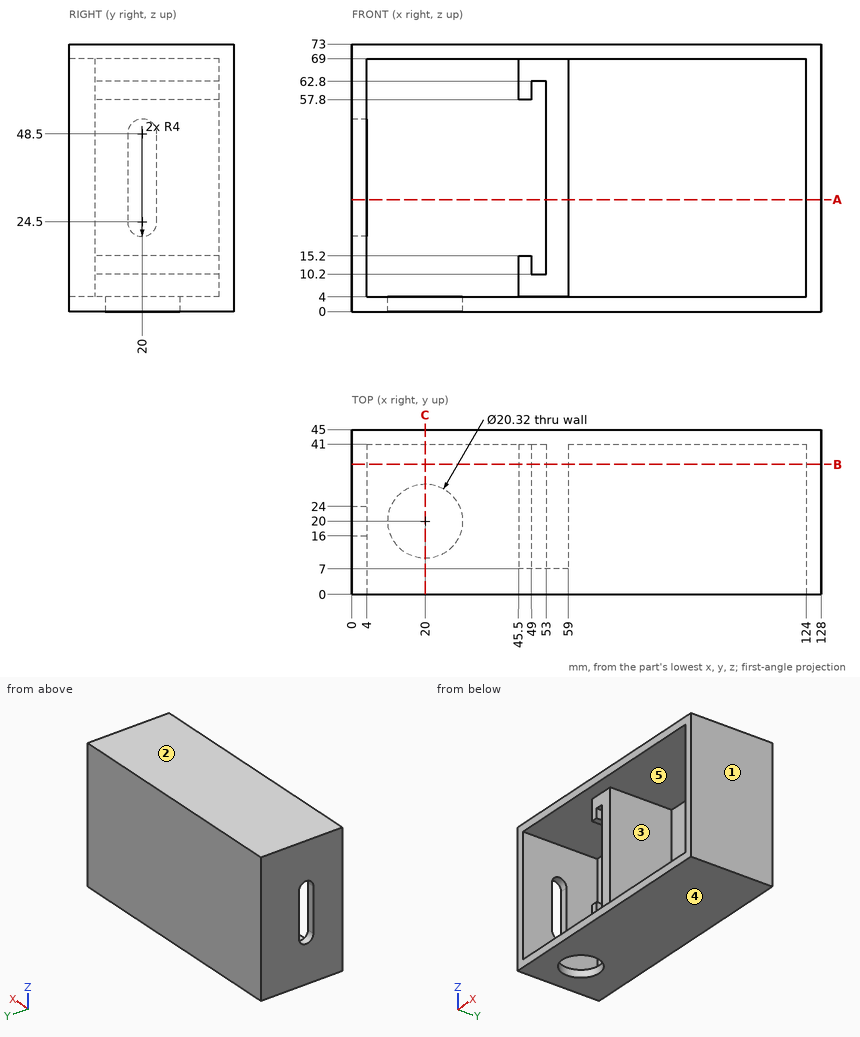
Answer from the drawing. Dimensions are ordinates in mm from the lowest x, y and z of the part. A direction names the side the tool comes from. Coordinates: 2 decimals unless noted, no trailing zeros. Loops run counter-clockwise (first coordinate to the right, second up) from the corner with the lowest first, then second, coordinate; pieces in that order, holes last. Notation, with made-up numbers: (-29.75, -30.5) -> (11.25, -30.5) arc R10 cw to (11.25, -24.5) -> close; hole circle Ø4 at (84, -21). An arc over 180 degrees is marked (long way). Answer in a Markdown table with one row per item.
Item 1: A cutting plane is placed at B-B on y = 35.5. Determine the outline of the cut face in (x, z).
Returned:
| item | result |
|---|---|
| outline | (0, 0) -> (128, 0) -> (128, 73) -> (0, 73) -> close; hole (4, 4) -> (45.5, 4) -> (45.5, 15.2) -> (49, 15.2) -> (49, 10.2) -> (53, 10.2) -> (53, 62.8) -> (49, 62.8) -> (49, 57.8) -> (45.5, 57.8) -> (45.5, 69) -> (4, 69) -> close; hole (59, 4) -> (124, 4) -> (124, 69) -> (59, 69) -> close |
Item 2: A cutting plane is placed at A-A on z = 30.5. Determine the outline of the cut face in (x, y).
Returned:
| item | result |
|---|---|
| outline | (0, 0) -> (4, 0) -> (4, 16) -> (0, 16) -> close; (0, 24) -> (4, 24) -> (4, 41) -> (53, 41) -> (53, 7) -> (59, 7) -> (59, 41) -> (124, 41) -> (124, 0) -> (128, 0) -> (128, 45) -> (0, 45) -> close |
Item 3: A cutting plane is placed at C-C on x = 20. Determine the outline of the cut face in (y, z), plus the area to 3 significant figures.
Returned:
| item | result |
|---|---|
| outline | (0, 0) -> (9.84, 0) -> (9.84, 4) -> (0, 4) -> close; (0, 69) -> (41, 69) -> (41, 4) -> (30.16, 4) -> (30.16, 0) -> (45, 0) -> (45, 73) -> (0, 73) -> close |
| area | 539 mm^2 |
Item 4: Each of these flat-tipped pins is pushed along its axis until it touches: P1, Ø11, axis at x = 52.5, z = 23.5, coming from the -Y side; P2, Ø6, axis at x = 92.5, z = 48.5, coming from the -Y side. Where does it stop, or does it pass through?
Returned:
| item | result |
|---|---|
| P1 | stops at y = 7 |
| P2 | stops at y = 41 |
Item 5: Straight lines are drawn through the part: line 1 along X through (y, z) = (9.5, 21.5); line 2 along Y through (x, z) = (20, 1.5); line 3 along X through (y, z) = (6.5, 63.5). For each, find the intervals that lie inside material, in ascending order. Write a range as [from, to].
Returned:
| item | result |
|---|---|
| line 1 | x = [0, 4], [53, 59], [124, 128] |
| line 2 | y = [0, 9.84], [30.16, 45] |
| line 3 | x = [0, 4], [124, 128] |
Item 6: For a pull along Z with two mould halves and no side action, classify the marked faces 1, 2 and 3 as released by +Z, released by -Z, zero draft, split by the parting line, or undercut.
Returned:
| item | result |
|---|---|
| face 1 | zero draft |
| face 2 | released by +Z |
| face 3 | undercut |
Item 7: For the marked faces 4 and 5, determine the directions among +Z, -Z, +X, -X, +Y, -Y from which every point of the face is accessible in a straight line to the end or side of a thin tool.
Returned:
| item | result |
|---|---|
| face 4 | -Z, +X, -X, +Y, -Y |
| face 5 | -Y |
